Verification items for the finished model (mm, model axes). A direction names the side the tool comes from. Round coordinates to 2 decimals unless told otherwise and drop trailing zeros. Write each loop counter-clockwise with the first axis right and the second up, starting at its lowest first coordinate (ties: lowest second). Pieces come first, ordered by that corner, then holes.
from build123d import *

# Parameters (mm, degrees)
SKETCH1_W               = 44.1
SKETCH1_H               = 32.5
BOSS_EXTRUDE1_DEPTH     = 25
SKETCH2_W               = 44.1
SKETCH2_H               = 26.75
CUT_EXTRUDE1_DEPTH      = 10
FILLET1_R               = 2
CUT_EXTRUDE2_DEPTH      = 38.084565523
CUT_EXTRUDE2_DEPTH_BACK = 38.084565523
SKETCH6_W               = 20
SKETCH6_H               = 3
SKETCH6_W_2             = 6
SKETCH6_H_2             = 2
SKETCH7_W               = 40.1
SKETCH7_H               = 1.25
CUT_EXTRUDE3_DEPTH      = 5.5
SKETCH8_W               = 0.85
SKETCH8_H               = 6
BOSS_EXTRUDE3_DEPTH     = 0.8
SKETCH9_R               = 1.35
CUT_EXTRUDE4_DEPTH      = 4
SKETCH11_W              = 40.1
SKETCH11_H              = 1.2
CUT_EXTRUDE5_DEPTH      = 0.8
SKETCH12_W              = 40.1
SKETCH12_H              = 1.2
CUT_EXTRUDE6_DEPTH      = 0.8
SKETCH13_W              = 35
SKETCH13_H              = 0.1
CUT_EXTRUDE8_DEPTH      = 47.555907251
SKETCH14_W              = 35
SKETCH14_H              = 4
BOSS_EXTRUDE4_DEPTH     = 32
SKETCH15_R              = 1.725
BOSS_EXTRUDE5_DEPTH     = 2.5
SKETCH16_W              = 40.1
SKETCH16_H              = 1.5
CUT_EXTRUDE9_DEPTH      = 5


with BuildPart() as part:
    # Sketch1 → Boss-Extrude1 (new body)
    with BuildSketch(Plane(origin=(0, 0, 0), x_dir=(1, 0, 0), z_dir=(0, 1, 0))):
        Rectangle(SKETCH1_W, SKETCH1_H)
    extrude(amount=BOSS_EXTRUDE1_DEPTH)

    # Sketch2 → Cut-Extrude1 (cut)
    with BuildSketch(Plane.XZ):
        Rectangle(SKETCH2_W, SKETCH2_H)
    extrude(amount=-CUT_EXTRUDE1_DEPTH, mode=Mode.SUBTRACT)

    # Fillet1
    fillet1_edges = [part.edges().sort_by_distance(p)[0] for p in [
        (-22.05, 25, 0),
        (0, 25, 16.25),
        (22.05, 25, 0),
        (0, 0, 16.25),
        (0, 0, -16.25),
        (22.05, 12.5, 16.25),
        (-22.05, 12.5, 16.25),
        (-22.05, 12.5, -16.25),
        (22.05, 12.5, -16.25),
        (0, 25, -16.25),
    ]]
    fillet(fillet1_edges, radius=FILLET1_R)

    # Sketch6 → Cut-Extrude2 (cut, two sides: drawn at the far end of the back side and taken through both)
    with BuildSketch(Plane(origin=(0, 0, 0), x_dir=(0, 0, -1), z_dir=(1, 0, 0)).offset(-CUT_EXTRUDE2_DEPTH_BACK)):
        with Locations((0, 12.1)):
            Rectangle(SKETCH6_W, SKETCH6_H)
        with Locations((0, 24)):
            Rectangle(SKETCH6_W_2, SKETCH6_H_2)
    extrude(amount=CUT_EXTRUDE2_DEPTH + CUT_EXTRUDE2_DEPTH_BACK, mode=Mode.SUBTRACT)

    # Sketch7 → Cut-Extrude3 (cut)
    with BuildSketch(Plane(origin=(0, 25, 0), x_dir=(1, 0, 0), z_dir=(0, 1, 0))):
        with Locations((0, 4.425)):
            Rectangle(SKETCH7_W, SKETCH7_H)
        with Locations((0, -4.425)):
            Rectangle(SKETCH7_W, SKETCH7_H)
    extrude(amount=-CUT_EXTRUDE3_DEPTH, mode=Mode.SUBTRACT)

    # Sketch8 → Boss-Extrude3 (add)
    with BuildSketch(Plane(origin=(0, 23, 0), x_dir=(1, 0, 0), z_dir=(0, 1, 0))):
        with Locations((-21.625, 0)):
            Rectangle(SKETCH8_W, SKETCH8_H)
        with Locations((21.625, 0)):
            Rectangle(SKETCH8_W, SKETCH8_H)
        with Locations((-19.625, 0)):
            Rectangle(SKETCH8_W, SKETCH8_H)
        with Locations((19.625, 0)):
            Rectangle(SKETCH8_W, SKETCH8_H)
        with Locations((-17.625, 0)):
            Rectangle(SKETCH8_W, SKETCH8_H)
        with Locations((17.625, 0)):
            Rectangle(SKETCH8_W, SKETCH8_H)
        with Locations((15.625, 0)):
            Rectangle(SKETCH8_W, SKETCH8_H)
        with Locations((-15.625, 0)):
            Rectangle(SKETCH8_W, SKETCH8_H)
        with Locations((13.625, 0)):
            Rectangle(SKETCH8_W, SKETCH8_H)
        with Locations((-13.625, 0)):
            Rectangle(SKETCH8_W, SKETCH8_H)
        with Locations((11.625, 0)):
            Rectangle(SKETCH8_W, SKETCH8_H)
        with Locations((-11.625, 0)):
            Rectangle(SKETCH8_W, SKETCH8_H)
        with Locations((9.625, 0)):
            Rectangle(SKETCH8_W, SKETCH8_H)
        with Locations((-9.625, 0)):
            Rectangle(SKETCH8_W, SKETCH8_H)
        with Locations((7.625, 0)):
            Rectangle(SKETCH8_W, SKETCH8_H)
        with Locations((-7.625, 0)):
            Rectangle(SKETCH8_W, SKETCH8_H)
    extrude(amount=BOSS_EXTRUDE3_DEPTH)

    # Sketch9 → Cut-Extrude4 (cut)
    with BuildSketch(Plane(origin=(0, 23, 0), x_dir=(1, 0, 0), z_dir=(0, 1, 0))):
        with Locations(Location((0, 0, 0), (0, 0, 270))):
            Circle(SKETCH9_R)
    extrude(amount=-CUT_EXTRUDE4_DEPTH, mode=Mode.SUBTRACT)

    # Sketch11 → Cut-Extrude5 (cut)
    with BuildSketch(Plane(origin=(0, 0, 3), x_dir=(-1, 0, 0), z_dir=(0, 0, -1))):
        with Locations((0, 24.4)):
            Rectangle(SKETCH11_W, SKETCH11_H)
    extrude(amount=-CUT_EXTRUDE5_DEPTH, mode=Mode.SUBTRACT)

    # Sketch12 → Cut-Extrude6 (cut)
    with BuildSketch(Plane.XY.offset(-3)):
        with Locations((0, 24.4)):
            Rectangle(SKETCH12_W, SKETCH12_H)
    extrude(amount=-CUT_EXTRUDE6_DEPTH, mode=Mode.SUBTRACT)

    # Sketch13 → Cut-Extrude8 (cut, through all)
    with BuildSketch(Plane(origin=(0, 0, -16.25), x_dir=(-1, 0, 0), z_dir=(0, 0, -1))):
        with Locations((-0.05, 21.95)):
            Rectangle(SKETCH13_W, SKETCH13_H)
    extrude(amount=-CUT_EXTRUDE8_DEPTH, mode=Mode.SUBTRACT)

    # Sketch14 → Boss-Extrude4 (add)
    with BuildSketch(Plane.XY.offset(16.25)):
        with Locations((0.05, 4)):
            Rectangle(SKETCH14_W, SKETCH14_H)
    extrude(amount=BOSS_EXTRUDE4_DEPTH)

    # Sketch15 → Boss-Extrude5 (add)
    with BuildSketch(Plane(origin=(0, 6, 0), x_dir=(1, 0, 0), z_dir=(0, 1, 0))):
        with Locations(Location((-13.45, -24.5, 0), (0, 0, 90))):
            Circle(SKETCH15_R)
        with Locations(Location((13.55, -24.5, 0), (0, 0, 90))):
            Circle(SKETCH15_R)
        with Locations(Location((13.55, -45, 0), (0, 0, 90))):
            Circle(SKETCH15_R)
        with Locations(Location((-13.45, -45, 0), (0, 0, 90))):
            Circle(SKETCH15_R)
    extrude(amount=BOSS_EXTRUDE5_DEPTH)

    # Sketch16 → Cut-Extrude9 (cut)
    with BuildSketch(Plane(origin=(0, 25, 0), x_dir=(1, 0, 0), z_dir=(0, 1, 0))):
        with Locations((0, 13.5)):
            Rectangle(SKETCH16_W, SKETCH16_H)
        with Locations((0, -13.5)):
            Rectangle(SKETCH16_W, SKETCH16_H)
    extrude(amount=-CUT_EXTRUDE9_DEPTH, mode=Mode.SUBTRACT)


solid = part.part
Q1. Depth check by flat-ended pin: P1, Ø0.9, axis at x = -12.5, y = 23, coming from the +Z side; P2, Ø0.5, axis at x = 21, y = 24.5, coming from the +Z side; P3, Ø10, axis at x = -8, z = 0, coming from the -Y side. Enter the tip coordinate at first touch or a pass-through.
Recorded:
P1: stops at z = 16.25
P2: stops at z = 15.54
P3: stops at y = 10
Q2. Material ranges on line 1 along Z through (x, y) = (-18, 21.5); line 2 along Z through (x, y) = (-19.5, 8.75) (3 decimals), recorded low to high.
Recorded:
line 1: z = -16.25 to -14.25, -12.75 to -5.05, -3.8 to 3.8, 5.05 to 12.75, 14.25 to 16.25
line 2: z = -16.25 to -13.375, 13.375 to 16.25
Q3. Sectioned sample at C-C (z = 11.5). Enter the section's corners in (x, y), plus the area to 3 significant figures.
Recorded:
outline: (-22.05, 10) - (22.05, 10) - (22.05, 23) arc R2 ccw to (20.05, 25) - (-20.05, 25) arc R2 ccw to (-22.05, 23) - close; hole (-17.45, 21.9) - (17.55, 21.9) - (17.55, 22) - (-17.45, 22) - close
area: 656 mm2
Q4. Sectioned sample at A-A (z = -8.5). Enter the section's corners in (x, y).
Recorded:
outline: (-22.05, 10) - (22.05, 10) - (22.05, 10.6) - (-22.05, 10.6) - close; (-22.05, 13.6) - (22.05, 13.6) - (22.05, 23) arc R2 ccw to (20.05, 25) - (-20.05, 25) arc R2 ccw to (-22.05, 23) - close; hole (-17.45, 21.9) - (17.55, 21.9) - (17.55, 22) - (-17.45, 22) - close
Q5. Tool access check on faces 4 (the flat face through (17.55, 4, 32)), 5 (the flat face through (0, 5, -13.375)), 6 (the flat face through (0, 23, -14.25)), 7 (the flat face through (0, 12, 10)). Record the directions out of +Z, -Z, +X, -X, +Y, -Y that give a thin tool (end or side, any length) a straight path to the whole face; none if there is none.
Recorded:
face 4: +Z, +X, +Y, -Y
face 5: +X, -X, -Y
face 6: +Y
face 7: +X, -X
Q6. Sectioned sample at D-D (y = 14.75). Enter the section's corners in (x, z).
Recorded:
outline: (-22.05, -14.25) arc R2 ccw to (-20.05, -16.25) - (20.05, -16.25) arc R2 ccw to (22.05, -14.25) - (22.05, 14.25) arc R2 ccw to (20.05, 16.25) - (-20.05, 16.25) arc R2 ccw to (-22.05, 14.25) - close
Q7. Release check for a two-part mould opening along X. For faces 1 (the flat face through (0, 5, 13.375)), 2 (the cylindrical face through (-11.766, 7.232, 45.374)), 3 (the flat face through (22.05, 17, 0)) record: released by +X, released by -X, zero draft, split by the parting line, or undercut.
Recorded:
face 1: zero draft
face 2: undercut
face 3: released by +X
Q8. Sectioned sample at B-B (y = 3.5). Enter the section's corners in (x, z) (3 decimals).
Recorded:
outline: (-22.05, -14.25) arc R2 ccw to (-20.05, -16.25) - (20.05, -16.25) arc R2 ccw to (22.05, -14.25) - (22.05, -13.375) - (-22.05, -13.375) - close; (-22.05, 13.375) - (22.05, 13.375) - (22.05, 14.25) arc R2 ccw to (20.05, 16.25) - (17.55, 16.25) - (17.55, 48.25) - (-17.45, 48.25) - (-17.45, 16.25) - (-20.05, 16.25) arc R2 ccw to (-22.05, 14.25) - close
